```python
from build123d import *

# Parameters (mm, degrees)
BOSS_EXTRUDE1_DEPTH           = 100
SKETCH3_R                     = 17.5
BOSS_EXTRUDE3_DEPTH           = 10
BOSS_EXTRUDE3_DRAFT           = 25
BOSS_EXTRUDE3_PROFILE_2_DEPTH = 10
BOSS_EXTRUDE3_PROFILE_2_DRAFT = 25
SKETCH4_R                     = 18
CUT_EXTRUDE1_DEPTH            = 11
CUT_EXTRUDE1_DRAFT            = -25
CUT_EXTRUDE1_PROFILE_2_DEPTH  = 11
CUT_EXTRUDE1_PROFILE_2_DRAFT  = -25
SKETCH5_W                     = 40
SKETCH5_H                     = 40
CUT_EXTRUDE2_DEPTH            = 144
SKETCH6_R                     = 85
CUT_EXTRUDE3_DEPTH            = 10
CUT_EXTRUDE4_START            = -10
SKETCH7_R                     = 85
CUT_EXTRUDE4_DEPTH            = 10
CUT_EXTRUDE5_DEPTH            = 10
CUT_EXTRUDE6_START            = -10
CUT_EXTRUDE6_DEPTH            = 10


with BuildPart() as part:
    # Sketch1 → Boss-Extrude1 (new body)
    with BuildSketch(Plane(origin=(0, 0, 0), x_dir=(1, 0, 0), z_dir=(0, 1, 0))):
        with BuildLine():
            Line((0, 150), (0, 75))
            ThreePointArc((0, 75), (53.033008589, 53.033008589), (75, 0))
            Line((75, 0), (150, 0))
            ThreePointArc((150, 0), (106.066017178, 106.066017178), (0, 150))
        make_face()
    extrude(amount=BOSS_EXTRUDE1_DEPTH)


with BuildPart() as boss_extrude3_tool:
    # Sketch3 → Boss-Extrude3 (with draft: the straight prism first)
    with BuildSketch(Plane(origin=(0, 110, 0), x_dir=(1, 0, 0), z_dir=(0, 1, 0))):
        with Locations((43.051886141, 103.936447408)):
            Circle(SKETCH3_R)
    extrude(amount=-BOSS_EXTRUDE3_DEPTH)
    # Boss-Extrude3: the draft: its side faces are tilted about the plane it starts from
    boss_extrude3_sides = [boss_extrude3_tool.faces().sort_by_distance(p)[0] for p in [
        (25.551886141, 105, -103.936447408),
    ]]
    draft(boss_extrude3_sides, Plane(origin=(0, 110, 0), x_dir=(1, 0, 0), z_dir=(0, 1, 0)), BOSS_EXTRUDE3_DRAFT)


with BuildPart() as part_1:
    add(part.part)

    # Boss-Extrude3: add boss_extrude3_tool
    add(boss_extrude3_tool.part)


with BuildPart() as boss_extrude3_profile_2_tool:
    # Sketch3 → Boss-Extrude3 profile 2 (with draft: the straight prism first)
    with BuildSketch(Plane(origin=(0, 110, 0), x_dir=(1, 0, 0), z_dir=(0, 1, 0))):
        with Locations((103.936447408, 43.051886141)):
            Circle(SKETCH3_R)
    extrude(amount=-BOSS_EXTRUDE3_PROFILE_2_DEPTH)
    # Boss-Extrude3 profile 2: the draft: its side faces are tilted about the plane it starts from
    boss_extrude3_profile_2_sides = [boss_extrude3_profile_2_tool.faces().sort_by_distance(p)[0] for p in [
        (86.436447408, 105, -43.051886141),
    ]]
    draft(boss_extrude3_profile_2_sides, Plane(origin=(0, 110, 0), x_dir=(1, 0, 0), z_dir=(0, 1, 0)), BOSS_EXTRUDE3_PROFILE_2_DRAFT)


with BuildPart() as part_2:
    add(part_1.part)

    # Boss-Extrude3 profile 2: add boss_extrude3_profile_2_tool
    add(boss_extrude3_profile_2_tool.part)


with BuildPart() as cut_extrude1_tool:
    # Sketch4 → Cut-Extrude1 (with draft: the straight prism first)
    with BuildSketch(Plane.XZ):
        with Locations((103.936447408, -43.051886141)):
            Circle(SKETCH4_R)
    extrude(amount=-CUT_EXTRUDE1_DEPTH)
    # Cut-Extrude1: the draft: its side faces are tilted about the plane it starts from
    cut_extrude1_sides = [cut_extrude1_tool.faces().sort_by_distance(p)[0] for p in [
        (85.936447408, 5.5, -43.051886141),
    ]]
    draft(cut_extrude1_sides, Plane.XZ, CUT_EXTRUDE1_DRAFT)


with BuildPart() as part_3:
    add(part_2.part)

    # Cut-Extrude1: cut by cut_extrude1_tool
    add(cut_extrude1_tool.part, mode=Mode.SUBTRACT)


with BuildPart() as cut_extrude1_profile_2_tool:
    # Sketch4 → Cut-Extrude1 profile 2 (with draft: the straight prism first)
    with BuildSketch(Plane.XZ):
        with Locations((43.051886141, -103.936447408)):
            Circle(SKETCH4_R)
    extrude(amount=-CUT_EXTRUDE1_PROFILE_2_DEPTH)
    # Cut-Extrude1 profile 2: the draft: its side faces are tilted about the plane it starts from
    cut_extrude1_profile_2_sides = [cut_extrude1_profile_2_tool.faces().sort_by_distance(p)[0] for p in [
        (25.051886141, 5.5, -103.936447408),
    ]]
    draft(cut_extrude1_profile_2_sides, Plane.XZ, CUT_EXTRUDE1_PROFILE_2_DRAFT)


with BuildPart() as part_4:
    add(part_3.part)

    # Cut-Extrude1 profile 2: cut by cut_extrude1_profile_2_tool
    add(cut_extrude1_profile_2_tool.part, mode=Mode.SUBTRACT)

    # Sketch5 → Cut-Extrude2 (cut)
    with BuildSketch(Plane.XZ):
        with Locations((0, -75)):
            Rectangle(SKETCH5_W, SKETCH5_H)
        with Locations((75, 0)):
            Rectangle(SKETCH5_W, SKETCH5_H)
    extrude(amount=-CUT_EXTRUDE2_DEPTH, mode=Mode.SUBTRACT)

    # Chamfer1
    # the kernel refuses this chamfer: 5 mm, written as the material it takes off along each edge
    with BuildSketch(Plane(origin=(0, 100, 0), x_dir=(0.9963251041879452, 0, 0.08565212644692502), z_dir=(-0.08565212644692502, 0, 0.9963251041879452))) as chamfer1_piece_1:
        with BuildLine():
            Line((150.141421356, -5.141421356), (144.858578644, 0.141421356))
            Line((144.858578644, 0.141421356), (144.858578644, 0.241421356))
            ThreePointArc((144.858578644, 0.241421356), (147.429289322, 0.1), (150, 0.1))
            Line((150, 0.1), (150.1, 0))
            ThreePointArc((150.1, 0), (150.1, -2.570710678), (150.241421356, -5.141421356))
            Line((150.241421356, -5.141421356), (150.141421356, -5.141421356))
        make_face()
    revolve(axis=Axis((0, 100, 0), (0, 1, 0)), revolution_arc=99.827051452, mode=Mode.SUBTRACT)
    with BuildSketch(Plane(origin=(0, 0, 0), x_dir=(0.9963251041879452, 0, 0.08565212644692488), z_dir=(-0.08565212644692488, 0, 0.9963251041879452))) as chamfer1_piece_2:
        with BuildLine():
            Line((150.141421356, 5.141421356), (144.858578644, -0.141421356))
            Line((144.858578644, -0.141421356), (144.858578644, -0.241421356))
            ThreePointArc((144.858578644, -0.241421356), (147.429289322, -0.1), (150, -0.1))
            Line((150, -0.1), (150.1, 0))
            ThreePointArc((150.1, 0), (150.1, 2.570710678), (150.241421356, 5.141421356))
            Line((150.241421356, 5.141421356), (150.141421356, 5.141421356))
        make_face()
    revolve(axis=Axis((0, 0, 0), (0, 1, 0)), revolution_arc=99.827051452, mode=Mode.SUBTRACT)
    with BuildSketch(Plane(origin=(150, -13.291214034, 0), x_dir=(0.009358737420086232, 0, -0.9999562060579963), z_dir=(0, 1, 0))) as chamfer1_piece_3:
        with BuildLine():
            Line((5.316485613, 0), (-0.192733912, 5.223619222))
            Line((-0.192733912, 5.223619222), (-0.292729532, 5.222683348))
            ThreePointArc((-0.292729532, 5.222683348), (-0.124446231, 2.611546813), (-0.099995621, -0.000935874))
            Line((-0.099995621, -0.000935874), (0.000935874, -0.099995621))
            ThreePointArc((0.000935874, -0.099995621), (2.659639048, -0.051556934), (5.320869055, -0.099903881))
            Line((5.320869055, -0.099903881), (5.316485613, 0))
        make_face()
    extrude(amount=126.582428067, mode=Mode.SUBTRACT)
    with BuildSketch(Plane(origin=(0, -13.291214034, -150), x_dir=(0.9999562060579963, 0, -0.009358737420086213), z_dir=(0, 1, 0))) as chamfer1_piece_4:
        with BuildLine():
            Line((5.316485613, 0), (-0.192733912, -5.223619222))
            Line((-0.192733912, -5.223619222), (-0.292729532, -5.222683348))
            ThreePointArc((-0.292729532, -5.222683348), (-0.124446231, -2.611546813), (-0.099995621, 0.000935874))
            Line((-0.099995621, 0.000935874), (0.000935874, 0.099995621))
            ThreePointArc((0.000935874, 0.099995621), (2.659639048, 0.051556934), (5.320869055, 0.099903881))
            Line((5.320869055, 0.099903881), (5.316485613, 0))
        make_face()
    extrude(amount=126.582428067, mode=Mode.SUBTRACT)

    # Sketch6 → Cut-Extrude3 (cut)
    with BuildSketch(Plane(origin=(0, 100, 0), x_dir=(1, 0, 0), z_dir=(0, 1, 0))):
        Circle(SKETCH6_R)
    extrude(amount=-CUT_EXTRUDE3_DEPTH, mode=Mode.SUBTRACT)

    # Sketch7 → Cut-Extrude4 (cut)
    with BuildSketch(Plane.XZ.offset(CUT_EXTRUDE4_START)):
        Circle(SKETCH7_R)
    extrude(amount=CUT_EXTRUDE4_DEPTH, mode=Mode.SUBTRACT)

    # Sketch8 → Cut-Extrude5 (cut)
    with BuildSketch(Plane(origin=(0, 100, 0), x_dir=(1, 0, 0), z_dir=(0, 1, 0))):
        with BuildLine():
            Line((66.757749743, 52.61561412), (86.620580695, 72.478445072))
            ThreePointArc((86.620580695, 72.478445072), (86.620580695, 86.620580695), (72.478445072, 86.620580695))
            Line((72.478445072, 86.620580695), (52.61561412, 66.757749743))
            ThreePointArc((52.61561412, 66.757749743), (60.104076401, 60.104076401), (66.757749743, 52.61561412))
        make_face()
    extrude(amount=-CUT_EXTRUDE5_DEPTH, mode=Mode.SUBTRACT)

    # Sketch10 → Cut-Extrude6 (cut)
    with BuildSketch(Plane.XZ.offset(CUT_EXTRUDE6_START)):
        with BuildLine():
            Line((86.620580695, -72.478445072), (66.757749743, -52.61561412))
            ThreePointArc((66.757749743, -52.61561412), (60.104076401, -60.104076401), (52.61561412, -66.757749743))
            Line((52.61561412, -66.757749743), (72.478445072, -86.620580695))
            ThreePointArc((72.478445072, -86.620580695), (86.620580695, -86.620580695), (86.620580695, -72.478445072))
        make_face()
    extrude(amount=CUT_EXTRUDE6_DEPTH, mode=Mode.SUBTRACT)


solid = part_4.part
```
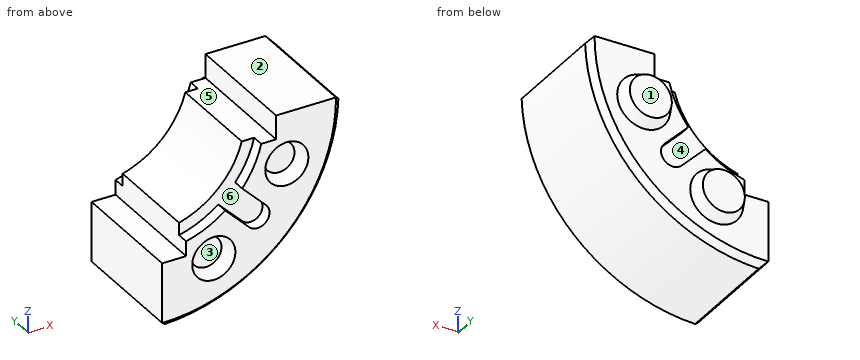
Verification items for the finished model (mm, model axes). Face numbers are marked on the shaded views. A direction names the side the tool comes from. Give positions to 0.01 mm unless a question says otherwise; leave off trailing zeros. Order: outer loops, then holes, each group sorted by start corner. A loop starts at its lowest first (then second) coordinate and runs counter-clockwise, first axis right, second up. Notation, with made-up numbers: (24, 84.25) - (58, 84.25) arc R4 cw to (58, 90.25) - close; hole circle Ø11 at (-25, -10). An arc over 180 degrees is marked (long way). Answer as CSV lines item,"result". Start each with the question number.
Item 1: Access from +Z, -Z, +X, -X, +Y, -Y to the whole of each face (thin tool, end or side, straight path). Record for the marked faces 4, 5 and 6.
Item 2: Gauge pin test, flat ends, axial feed: pin 1 (8 mm diameter, centred on y = 55.5, z = -24, fed in from +X); pin 2 (5 mm diameter, centred on x = 90, y = 61, fed in from +Z); pin 3 (16 mm diameter, centred on x = 7, y = 34, fed in from +Z); pin 4 (25 mm diameter, centred on y = 51, z = -86, fed in from -X). Record the tip position at first contact, or that the pin passes through.
Item 3: Material ranges on L1, parallel to Y at x = 92.5, z = -106.5; L2, parallel to Y at x = 32, z = -100.5; L3, parallel to Z at x = 83.5, y = 92, recorded low to high.
Item 4: Mould release check, pull along Z, two halves, no side actions. Record for the marked faces 1, 2 and 3: released by +Z, released by -Z, zero draft, split by the parting line, or undercut.
Item 5: Section check A-A, the plane y = 52. Record the boundary of the cut face in (x, z), plus the area to 3 significant figures.
Filled in:
1,face 4,"+Y"
1,face 5,"+Z, -X, +Y, -Y"
1,face 6,"-Y"
2,pin 1,"x = 148.66"
2,pin 2,"z = -20"
2,pin 3,"z = -95"
2,pin 4,"x = 0"
3,L1,"0 to 100"
3,L2,"11 to 110"
3,L3,"-124.61 to -88.74, -69.36 to -20"
4,face 1,"zero draft"
4,face 2,"released by +Z"
4,face 3,"undercut"
5,outline,"(0, -144.91) - (5.17, -149.91) arc R150 ccw to (149.91, -5.17) - (144.91, 0) - (95, 0) - (95, -20) - (72.28, -20) arc R75 cw to (20, -72.28) - (20, -95) - (0, -95) - close"
5,area,"12,400 mm^2"
